```python
from build123d import *
from build123d.topology import SkipClean

# Parameters (mm, degrees)
SKETCH_1_R          = 1.05
EXTRUDE_1_DEPTH     = 2.5
SKETCH_2_W          = 82
SKETCH_2_H          = 7
CUT_EXTRUDE_1_DEPTH = 2.5
SKETCH_3_W          = 79
SKETCH_3_H          = 4
EXTRUDE_2_DEPTH     = 10.7
SKETCH_4_W          = 0.401921616
SKETCH_4_H          = 13.2
EXTRUDE_3_DEPTH     = 0.6
SKETCH_5_W          = 6.198078384
SKETCH_5_H          = 0.4
EXTRUDE_4_DEPTH     = 0.4
SKETCH_6_W          = 79
SKETCH_6_H          = 6.717043916
CUT_EXTRUDE_2_DEPTH = 20
EXTRUDE_START       = 2.5
SKETCH_7_R          = 1.05
EXTRUDE_5_DEPTH     = 2.5
SKETCH_9_R          = 1
CUT_EXTRUDE_3_DEPTH = 10
SKETCH_10_R         = 1
CUT_EXTRUDE_4_DEPTH = 10
SKETCH_11_W         = 5
SKETCH_11_H         = 9.9
CUT_EXTRUDE_5_DEPTH = 28
SKETCH_13_R         = 8.45
SKETCH_13_R_2       = 1.05
EXTRUDE_7_DEPTH     = 2


with BuildPart() as part:
    # Sketch 1 → Extrude 1 (new body)
    with BuildSketch(Plane.XY):
        with BuildLine():
            Line((0, 8.45), (110, 8.45))
            Line((110, 8.45), (110, -8.45))
            Line((110, -8.45), (0, -8.45))
            ThreePointArc((0, -8.45), (-8.45, 0), (0, 8.45))
        make_face()
        with Locations((-5.95, 0)):
            Circle(SKETCH_1_R, mode=Mode.SUBTRACT)
        with Locations((0, 5.95)):
            Circle(SKETCH_1_R, mode=Mode.SUBTRACT)
        with Locations((5.95, 0)):
            Circle(SKETCH_1_R, mode=Mode.SUBTRACT)
        with Locations((0, -5.95)):
            Circle(SKETCH_1_R, mode=Mode.SUBTRACT)
    extrude(amount=EXTRUDE_1_DEPTH)

    # Sketch 2 → Cut-Extrude 1 (cut)
    with BuildSketch(Plane(origin=(0, 0, 0), x_dir=(-1, 0, 0), z_dir=(0, 0, -1))):
        with Locations((-69, -4.95)):
            Rectangle(SKETCH_2_W, SKETCH_2_H)
    extrude(amount=-CUT_EXTRUDE_1_DEPTH, mode=Mode.SUBTRACT)

    # Sketch 3 → Extrude 2 (add)
    with BuildSketch(Plane(origin=(0, 0, 0), x_dir=(-1, 0, 0), z_dir=(0, 0, -1))):
        with Locations((-67.5, 0.55)):
            Rectangle(SKETCH_3_W, SKETCH_3_H)
    extrude(amount=EXTRUDE_2_DEPTH)

    # Sketch 4 → Extrude 3 (add)
    with BuildSketch(Plane.XZ.offset(1.45)):
        with Locations((74.1, -4.1)):
            Rectangle(SKETCH_4_W, SKETCH_4_H)
        with Locations((67.5, -4.1)):
            Rectangle(SKETCH_4_W, SKETCH_4_H)
        with Locations((80.7, -4.1)):
            Rectangle(SKETCH_4_W, SKETCH_4_H)
        with Locations((87.3, -4.1)):
            Rectangle(SKETCH_4_W, SKETCH_4_H)
        with Locations((93.9, -4.1)):
            Rectangle(SKETCH_4_W, SKETCH_4_H)
    extrude(amount=EXTRUDE_3_DEPTH)

    # Sketch 5 → Extrude 4 (add)
    with BuildSketch(Plane.XZ.offset(1.45)):
        with Locations((70.8, 0.95)):
            Rectangle(SKETCH_5_W, SKETCH_5_H)
        with Locations((70.8, -9.15)):
            Rectangle(SKETCH_5_W, SKETCH_5_H)
        with Locations((77.4, 0.95)):
            Rectangle(SKETCH_5_W, SKETCH_5_H)
        with Locations((77.4, -9.15)):
            Rectangle(SKETCH_5_W, SKETCH_5_H)
        with Locations((84, 0.95)):
            Rectangle(SKETCH_5_W, SKETCH_5_H)
        with Locations((84, -9.15)):
            Rectangle(SKETCH_5_W, SKETCH_5_H)
        with Locations((90.6, 0.95)):
            Rectangle(SKETCH_5_W, SKETCH_5_H)
        with Locations((90.6, -9.15)):
            Rectangle(SKETCH_5_W, SKETCH_5_H)
    extrude(amount=EXTRUDE_4_DEPTH)

    # Sketch 6 → Cut-Extrude 2 (cut)
    with BuildSketch(Plane(origin=(0, 0, -10.7), x_dir=(-1, 0, 0), z_dir=(0, 0, -1))):
        with Locations((-67.5, -0.808521958)):
            Rectangle(SKETCH_6_W, SKETCH_6_H)
    extrude(amount=-CUT_EXTRUDE_2_DEPTH, mode=Mode.SUBTRACT)

    # Sketch 7 → Extrude 5 (add)
    with SkipClean():  # the faces are left unmerged after this step: merging them gives an invalid solid
        with BuildSketch(Plane(origin=(0, 0, 0), x_dir=(-1, 0, 0), z_dir=(0, 0, -1)).offset(EXTRUDE_START)):
            with BuildLine():
                Line((-110, -1.45), (-107, -1.45))
                Line((-107, -1.45), (-107, 2.55))
                Line((-107, 2.55), (-28, 2.55))
                Line((-28, 2.55), (-28, -8.45))
                Line((-28, -8.45), (0, -8.45))
                ThreePointArc((0, -8.45), (8.45, 0), (0, 8.45))
                Line((0, 8.45), (-110, 8.45))
                Line((-110, 8.45), (-110, -1.45))
            make_face()
            with Locations((-5.95, 0)):
                Circle(SKETCH_7_R, mode=Mode.SUBTRACT)
            with Locations((5.95, 0)):
                Circle(SKETCH_7_R, mode=Mode.SUBTRACT)
            with Locations((0, 5.95)):
                Circle(SKETCH_7_R, mode=Mode.SUBTRACT)
            with Locations((0, -5.95)):
                Circle(SKETCH_7_R, mode=Mode.SUBTRACT)
        extrude(amount=-EXTRUDE_5_DEPTH)

    # Sketch 9 → Cut-Extrude 3 (cut)
    with SkipClean():  # the faces are left unmerged after this step: merging them gives an invalid solid
        with BuildSketch(Plane.XZ.offset(-2.55)):
            with Locations(Location((102, 0, 0), (0, 0, 270))):
                Circle(SKETCH_9_R)
            with Locations(Location((33, 0, 0), (0, 0, 270))):
                Circle(SKETCH_9_R)
        extrude(amount=-CUT_EXTRUDE_3_DEPTH, mode=Mode.SUBTRACT)

    # Sketch 10 → Cut-Extrude 4 (cut)
    with SkipClean():  # the faces are left unmerged after this step: merging them gives an invalid solid
        with BuildSketch(Plane.XZ.offset(-2.55)):
            with Locations(Location((77.5, 0, 0), (0, 0, 270))):
                Circle(SKETCH_10_R)
        extrude(amount=-CUT_EXTRUDE_4_DEPTH, mode=Mode.SUBTRACT)

    # Sketch 11 → Cut-Extrude 5 (cut)
    with SkipClean():  # the faces are left unmerged after this step: merging them gives an invalid solid
        with BuildSketch(Plane(origin=(110, 0, 0), x_dir=(0, 0, -1), z_dir=(1, 0, 0))):
            with Locations((0, 3.5)):
                Rectangle(SKETCH_11_W, SKETCH_11_H)
        extrude(amount=-CUT_EXTRUDE_5_DEPTH, mode=Mode.SUBTRACT)

    # Sketch 13 → Extrude 7 (add)
    with SkipClean():  # the faces are left unmerged after this step: merging them gives an invalid solid
        with BuildSketch(Plane.XY.offset(2.5)):
            with Locations(Location((0, 0, 0), (0, 0, 90))):
                Circle(SKETCH_13_R)
            with Locations(Location((0, -5.95, 0), (0, 0, 180))):
                Circle(SKETCH_13_R_2, mode=Mode.SUBTRACT)
            with Locations(Location((5.95, 0, 0), (0, 0, 180))):
                Circle(SKETCH_13_R_2, mode=Mode.SUBTRACT)
            with Locations(Location((0, 5.95, 0), (0, 0, 180))):
                Circle(SKETCH_13_R_2, mode=Mode.SUBTRACT)
            with Locations(Location((-5.95, 0, 0), (0, 0, 180))):
                Circle(SKETCH_13_R_2, mode=Mode.SUBTRACT)
        extrude(amount=EXTRUDE_7_DEPTH)
    add(part.part.scale(1), mode=Mode.REPLACE)  # the faces are merged on a copy


solid = part.part
```
Check sheet for the modelled part. Datum: model origin and axes. Units: mm. Round coordinates to 2 decimals unless told otherwise and drop trailing zeros. Loops run counter-clockwise (first coordinate to the right, second up) from the corner with the lowest first, then second, coordinate; pieces in that order, holes last. Notation, with made-up numbers: M 20,-7.5 L 63,-7.5 A20 ccw 63,27.5 Z; hole C -32,-32.5 d4. An arc over 180 degrees is marked long. Answer as a JSON object with one key per item and string values.
1. Section check D-D (x = 77.5). Record the boundary of the cut face in (y, z), plus the area to 3 significant figures.
Reply:
{"outline": "M 2.55,-2.5 L 8.45,-2.5 L 8.45,-1 L 2.55,-1 Z; M 2.55,1 L 8.45,1 L 8.45,2.5 L 2.55,2.5 Z", "area": "17.7 mm²"}
2. Mould release check, pull along Z, two halves, no side actions. Record for faces 1 (the cylindrical face through (76.61, 5.46, -0.46)), 2 (the flat face through (82, 6, 0)), 3 (the flat face through (32, 4, 2.5)): pulls with the +Z half, pulls with the -Z half, needs draft (parallel to the pull), parting line crosses it, or undercut.
Reply:
{"face 1": "undercut", "face 2": "needs draft", "face 3": "pulls with the +Z half"}
3. Section check A-A (x = 5.95). Record the boundary of the cut face in (y, z), plus the area to 3 significant figures.
Reply:
{"outline": "M -8.45,-2.5 L -1.05,-2.5 L -1.05,4.5 L -6,4.5 L -6,2.5 L -8.45,2.5 Z; M 1.05,-2.5 L 8.45,-2.5 L 8.45,2.5 L 6,2.5 L 6,4.5 L 1.05,4.5 Z", "area": "93.8 mm²"}
4. Section check C-C (z = 3.5). Record the boundary of the cut face in (x, y).
Reply:
{"outline": "C 0,0 d16.9; hole C -5.95,0 d2.1; hole C 0,-5.95 d2.1; hole C 0,5.95 d2.1; hole C 5.95,0 d2.1"}
5. Scan lines: line 1 (X direction, y = 0, z = 0.75); line 2 (Y direction, x = 5.95, z = -1.05); line 3 (X direction, y = 5.5, z = 0.5). Record each from-to range of solid material in increasing order.
Reply:
{"line 1": "x = -8.45 to -7, -4.9 to 4.9, 7 to 28", "line 2": "y = -8.45 to -1.05, 1.05 to 8.45", "line 3": "x = -6.42 to -0.95, 0.95 to 32.13, 33.87 to 76.63, 78.37 to 82"}
6. Gauge pin test, flat ends, axial feed: P1, Ø1.7, axis at x = 5.95, y = 0, coming from the -Z side; P2, Ø2, axis at y = 2, z = 0.5, coming from the -X side; P3, Ø3, axis at x = 33, z = 0, coming from the -Y side; P4, Ø3, axis at y = -4.5, z = -1.5, coming from the +X side. Record the tip position at first contact, or that the pin passes through.
Reply:
{"P1": "passes through", "P2": "stops at x = -8.39", "P3": "stops at y = 2.55", "P4": "stops at x = 28"}
7. Section check B-B (y = -5.95). Record the boundary of the cut face in (x, z), plus the area to 3 significant figures.
Reply:
{"outline": "M -6,-2.5 L -1.05,-2.5 L -1.05,4.5 L -6,4.5 Z; M 1.05,-2.5 L 28,-2.5 L 28,2.5 L 6,2.5 L 6,4.5 L 1.05,4.5 Z", "area": "179 mm²"}
